Part model, mm, in its own coordinate system. Give positions to 0.01 mm unless a question says otherwise; leave off trailing zeros. Order: outer loops, then holes, each group sorted by start corner. A loop starts at its lowest first (then second) coordinate and runs counter-clockwise, first axis right, second up.
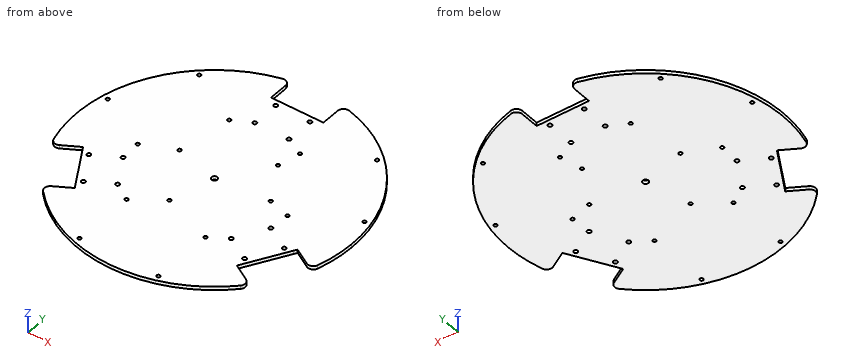
from build123d import *

# Parameters (mm, degrees)
SKETCH1_R           = 1.73
SKETCH1_R_2         = 2.5
BOSS_EXTRUDE2_DEPTH = 3
CUT_EXTRUDE1_DEPTH  = 10
SKETCH4_R           = 1.5
CUT_EXTRUDE2_DEPTH  = 153.155671711
BOSS_EXTRUDE3_DEPTH = 3
FILLET1_R           = 5
SKETCH6_R           = 1.5
CUT_EXTRUDE3_DEPTH  = 187.151001088


with BuildPart() as part:
    # Sketch1 → Boss-Extrude2 (new body)
    with BuildSketch(Plane.XY):
        Polygon((2.360735498, 103.328982943), (-74.24180488, -29.350508981), (-54.24180488, -63.991525133), (98.963275877, -63.991525133), (118.963275877, -29.350508981), (42.360735498, 103.328982943), align=None)
        with Locations((7.415735498, 93.328982943)):
            Circle(SKETCH1_R, mode=Mode.SUBTRACT)
        with Locations((37.305735498, 93.328982943)):
            Circle(SKETCH1_R, mode=Mode.SUBTRACT)
        with Locations((37.305735498, 69.268982943)):
            Circle(SKETCH1_R, mode=Mode.SUBTRACT)
        with Locations((7.415735498, 69.268982943)):
            Circle(SKETCH1_R, mode=Mode.SUBTRACT)
        with Locations((107.775521839, -28.728267397)):
            Circle(SKETCH1_R, mode=Mode.SUBTRACT)
        with Locations((86.938950624, -16.698267397)):
            Circle(SKETCH1_R, mode=Mode.SUBTRACT)
        with Locations((71.993950624, -42.583766716)):
            Circle(SKETCH1_R, mode=Mode.SUBTRACT)
        with Locations((92.830521839, -54.613766716)):
            Circle(SKETCH1_R, mode=Mode.SUBTRACT)
        with Locations((-42.217479627, -16.698267397)):
            Circle(SKETCH1_R, mode=Mode.SUBTRACT)
        with Locations((-27.272479627, -42.583766716)):
            Circle(SKETCH1_R, mode=Mode.SUBTRACT)
        with Locations((-63.054050843, -28.728267397)):
            Circle(SKETCH1_R, mode=Mode.SUBTRACT)
        with Locations((-48.109050843, -54.613766716)):
            Circle(SKETCH1_R, mode=Mode.SUBTRACT)
        with Locations((22.360735498, 3.328982943)):
            Circle(SKETCH1_R_2, mode=Mode.SUBTRACT)
    extrude(amount=BOSS_EXTRUDE2_DEPTH)

    # Sketch2 → Cut-Extrude1 (cut)
    with BuildSketch(Plane.XY.offset(3)):
        Polygon((-69.911677861, -26.850508981), (-71.355053534, -24.350508981), (-74.24180488, -29.350508981), align=None)
        Polygon((-48.468302188, -63.991525133), (-69.911677861, -26.850508981), (-74.24180488, -29.350508981), (-54.24180488, -63.991525133), align=None)
        Polygon((118.963275877, -29.350508981), (114.633148858, -26.850508981), (93.189773185, -63.991525133), (98.963275877, -63.991525133), align=None)
        Polygon((118.963275877, -29.350508981), (116.076524531, -24.350508981), (114.633148858, -26.850508981), align=None)
        Polygon((7.415735498, 98.328982943), (7.415735498, 103.328982943), (2.360735498, 103.328982943), (-0.526015848, 98.328982943), align=None)
        Polygon((42.360735498, 103.328982943), (7.415735498, 103.328982943), (7.415735498, 98.328982943), (45.247486844, 98.328982943), align=None)
    extrude(amount=-CUT_EXTRUDE1_DEPTH, mode=Mode.SUBTRACT)

    # Sketch4 → Cut-Extrude2 (cut, through all)
    with BuildSketch(Plane.XY.offset(3)):
        with Locations((12.112024192, -34.919728363)):
            Circle(SKETCH4_R)
        with Locations((68.733802457, 7.008474867)):
            Circle(SKETCH4_R)
        with Locations((48.733802457, 41.649491019)):
            Circle(SKETCH4_R)
        with Locations((-15.887975808, 13.577694249)):
            Circle(SKETCH4_R)
    extrude(amount=-CUT_EXTRUDE2_DEPTH, mode=Mode.SUBTRACT)

    # Sketch5 → Boss-Extrude3 (add)
    with BuildSketch(Plane.XY.offset(3)):
        with BuildLine():
            Line((45.247486844, 121.128982943), (45.247486844, 98.328982943))
            Line((45.247486844, 98.328982943), (116.076524531, -24.350508981))
            Line((116.076524531, -24.350508981), (135.821903737, -35.750508981))
            ThreePointArc((135.821903737, -35.750508981), (140.716740282, -16.482617667), (142.363416248, 3.328982943))
            ThreePointArc((142.363416248, 3.328982943), (114.954242026, 79.664334753), (45.247486844, 121.128982943))
        make_face()
        with BuildLine():
            Line((-71.355053534, -24.350508981), (-0.526015848, 98.328982943))
            Line((-0.526015848, 98.328982943), (-0.526015848, 121.128982943))
            ThreePointArc((-0.526015848, 121.128982943), (-81.564634554, 63.330323318), (-91.100432741, -35.750508981))
            Line((-91.100432741, -35.750508981), (-71.355053534, -24.350508981))
        make_face()
        with BuildLine():
            Line((93.189773185, -63.991525133), (-48.468302188, -63.991525133))
            Line((-48.468302188, -63.991525133), (-68.213681395, -75.391525133))
            ThreePointArc((-68.213681395, -75.391525133), (22.360735498, -116.673697807), (112.935152391, -75.391525133))
            Line((112.935152391, -75.391525133), (93.189773185, -63.991525133))
        make_face()
    extrude(amount=-BOSS_EXTRUDE3_DEPTH)

    # Fillet1
    fillet1_edges = [part.edges().sort_by_distance(p)[0] for p in [
        (135.821903737, -35.750508981, 1.5),
        (45.247486844, 121.128982943, 1.5),
        (-0.526015848, 121.128982943, 1.5),
        (-91.100432741, -35.750508981, 1.5),
        (-68.213681395, -75.391525133, 1.5),
        (112.935152391, -75.391525133, 1.5),
    ]]
    fillet(fillet1_edges, radius=FILLET1_R)

    # Sketch6 → Cut-Extrude3 (cut, through all)
    with BuildSketch(Plane(origin=(0, 0, 0), x_dir=(-1, 0, 0), z_dir=(0, 0, -1))):
        with BuildLine():
            ThreePointArc((91.295141666, 28.245040241), (90.545141666, 29.544078346), (89.045141666, 29.544078346))
            Line((89.045141666, 29.544078346), (89.795141666, 28.245040241))
            Line((89.795141666, 28.245040241), (88.49610356, 27.495040241))
            ThreePointArc((88.49610356, 27.495040241), (90.183370233, 26.796151501), (91.295141666, 28.245040241))
        make_face()
        with BuildLine():
            Line((89.795141666, 28.245040241), (89.045141666, 29.544078346))
            ThreePointArc((89.045141666, 29.544078346), (88.346252926, 28.633268808), (88.49610356, 27.495040241))
            Line((88.49610356, 27.495040241), (89.795141666, 28.245040241))
        make_face()
        with BuildLine():
            ThreePointArc((91.295141666, 28.245040241), (90.545141666, 29.544078346), (89.045141666, 29.544078346))
            Line((89.045141666, 29.544078346), (89.795141666, 28.245040241))
            Line((89.795141666, 28.245040241), (88.49610356, 27.495040241))
            ThreePointArc((88.49610356, 27.495040241), (90.183370233, 26.796151501), (91.295141666, 28.245040241))
        make_face()
        with BuildLine():
            Line((89.795141666, 28.245040241), (89.045141666, 29.544078346))
            ThreePointArc((89.045141666, 29.544078346), (88.346252926, 28.633268808), (88.49610356, 27.495040241))
            Line((88.49610356, 27.495040241), (89.795141666, 28.245040241))
        make_face()
        with Locations((43.029769861, 1.245040241)):
            Circle(SKETCH6_R)
        with Locations((8.529769861, 61.000793102)):
            Circle(SKETCH6_R)
        with Locations((55.295141666, 88.000793102)):
            Circle(SKETCH6_R)
        with Locations((-100.016612662, 88.000793102)):
            Circle(SKETCH6_R)
        with Locations((-53.251240857, 61.000793102)):
            Circle(SKETCH6_R)
        with Locations((-134.516612662, 28.245040241)):
            Circle(SKETCH6_R)
        with Locations((-87.751240857, 1.245040241)):
            Circle(SKETCH6_R)
        with Locations((-56.860735498, -52.258884513)):
            Circle(SKETCH6_R)
        with Locations((12.139264502, -52.258884513)):
            Circle(SKETCH6_R)
        with Locations((-56.860735498, -106.258884513)):
            Circle(SKETCH6_R)
        with Locations((12.139264502, -106.258884513)):
            Circle(SKETCH6_R)
    extrude(amount=-CUT_EXTRUDE3_DEPTH, mode=Mode.SUBTRACT)


solid = part.part
Item 1: Band-saw the part on B-B on y = -67. List the corners of the cut face in (x, z).
Item 2: Drop flat-ended pins along their axis: P1, Ø1, axis at x = 40.5, z = 0.5, coming from the -Y side; P2, Ø1.5, axis at y = 20.5, z = 2, coming from the +X side; P3, Ø1.5, axis at y = -29, z = 2.5, coming from the +X side. Give the stop position or say it passes through.
Item 3: Band-saw the part on A-A on z = 1.5. Give the number of separate pieces and of enclosed holes in the cut face, plus the area to 3 significant figures.
Item 4: Drill centre lines: probe 1 along Y at (x, z) = (-11.5, 1.8); probe 2 along X at (y, z) = (89, 2.85); probe 3 along Y at (x, z) = (-47, 2.7). Where is each one in solid material? Low to high.
Working result:
1. outline: (-53.68, 0) - (98.4, 0) - (98.4, 3) - (-53.68, 3) - close
2. P1: stops at y = -115.37
2. P2: stops at x = 141.23
2. P3: stops at x = 138.13
3. separate pieces: 1
3. enclosed holes: 29
3. area: 41,600 mm2
4. probe 1: y = -111.8 to -107.62, -104.9 to -53.62, -50.9 to 118.46
4. probe 2: x = -61.67 to -56.41, -54.18 to 98.9, 101.14 to 106.39
4. probe 3: y = -94.6 to -55.94, -53.29 to 101.26
